Read the model definition and answer for the solid it produces. Units are mm, in the model's axes. A direction names the side the tool comes from. Round coordinates to 2 decimals unless told otherwise and drop trailing zeros. One line per item, written item: value. Start each with the question number.
(1) The mould has two halves that part along Y. Classify faces 3 (the face through (0, -4, 20)), 4 (the face through (-5.5, 0, 12.7)), 5 (the face through (-3.47, -15.62, 4.06)): +Y half, -Y half, draft (parallel to the pull), parting line (faces both ways), or undercut.
(2) Flat-ended cylindrical pins translate along their axes: pin 1 Ø3 at (x, z) = (12.5, 8.5) entering from +Y; pin 2 Ø0.5 at (y, z) = (-0.5, 12) entering from -X; pin 3 Ø11.5 at (x, z) = (9.5, 12.5) entering from +Y; pin 4 Ø3 at (x, y) = (0, 0) entering from +Z. Find the tip coordinate at first contact, or state that the pin passes through.
(3) Find the intervals of material crossed by L1, parallel to Y at x = 0, z = 3.65; L2, parallel to Y at x = 7, z = 16.5; L3, parallel to X at y = -1, z = 14, in increasing order.
(4) For faces 1 (the face through (9, -0.6, 7)), 2 (the face through (4.4, -3.3, 12.7)), determine the directions among +Z, -Z, +X, -X, +Y, -Y from which every point of the face is accessible in a straight line to the end or side of a thin tool.
from build123d import *

# Parameters (mm, degrees)
PAD_DEPTH          = 0.6
POLARPATTERN_COUNT = 5


with BuildPart() as part:
    # Sketch → Revolution (revolve)
    with BuildSketch(Plane.XZ):
        with BuildLine():
            Line((16, 0), (16, 8))
            ThreePointArc((16, 8), (13.1723, 15.81025), (6, 20))
            Line((3.8, 20), (6, 20))
            Line((3.8, 8), (3.8, 20))
            Line((1.8, 6), (3.8, 8))
            Line((1.8, 6), (1.8, 0))
            Line((1.8, 0), (3.8, 0))
            Line((3.8, 0), (3.8, 5.5))
            Line((3.8, 5.5), (5.5, 7.2))
            Line((5.5, 7.2), (5.5, 18))
            ThreePointArc((14, 8), (11.587885, 14.562202), (5.5, 18))
            Line((14, 0), (14, 8))
            Line((16, 0), (14, 0))
        make_face()
    revolve(axis=Axis((0, 0, 0), (0, 0, 1)))

    # Sketch001 → Pad (new body, symmetric)
    with BuildSketch(Plane.XZ):
        with BuildLine():
            Line((14.5, 0), (14.5, 8))
            ThreePointArc((14.5, 8), (11.942101, 14.914658), (5.5, 18.5))
            Line((5.5, 7.5), (5.5, 18.5))
            Line((3.5, 5.5), (5.5, 7.5))
            Line((3.5, 0), (3.5, 5.5))
            Line((3.5, 0), (14.5, 0))
        make_face()
    pad = extrude(amount=PAD_DEPTH, both=True)

    # PolarPattern: Pad ×5 about axis
    polarpattern_axis = Axis((0, 0, 0), (0, 0, 1))
    for i in range(1, POLARPATTERN_COUNT):
        add(pad.rotate(polarpattern_axis, i * 360 / POLARPATTERN_COUNT))


solid = part.part
Here are the results:
1. face 3: draft
1. face 4: undercut
1. face 5: parting line
2. pin 1: y = 11.61
2. pin 2: x = -15.4
2. pin 3: y = 15.24
2. pin 4: through
3. L1: -16 to -14, -3.8 to -1.8, 1.8 to 3.8, 14 to 16
3. L2: -10.42 to -6.25, -0.6 to 0.6, 6.25 to 10.42
3. L3: -14.39 to -11.99, -5.41 to -3.67, 3.67 to 5.41, 11.99 to 14.39
4. face 1: -Z
4. face 2: none
